from build123d import *

# Parameters (mm, degrees)
SKETCH_R          = 11
PAD_DEPTH         = 5
SKETCH001_R       = 11
PAD001_DEPTH      = 3
SKETCH002_R       = 4.2
PAD002_DEPTH      = 8
SKETCH003_W       = 25.13587
SKETCH003_H       = 8
POCKET_DEPTH      = 11.001
POCKET_DEPTH_BACK = -11.001


with BuildPart() as part:
    # Sketch → Pad (new body)
    with BuildSketch(Plane.XY):
        Circle(SKETCH_R)
        with BuildLine():
            ThreePointArc((-2.683282, 3.1), (0, -4.1), (2.683282, 3.1))
            Line((2.683282, 3.1), (-2.683282, 3.1))
        make_face(mode=Mode.SUBTRACT)
    extrude(amount=-PAD_DEPTH)

    # Sketch001 → Pad001 (join)
    with BuildSketch(Plane.XY.offset(3)):
        Circle(SKETCH001_R)
    extrude(amount=-PAD001_DEPTH)

    # Sketch002 → Pad002 (join)
    with BuildSketch(Plane.XY.offset(11)):
        with Locations((0, 4)):
            Circle(SKETCH002_R)
    extrude(amount=-PAD002_DEPTH)

    # Sketch003 → Pocket (cut, two sides)
    with BuildSketch(Plane.XZ) as pocket_sk:
        with Locations((0.504129, -1)):
            Rectangle(SKETCH003_W, SKETCH003_H)
    extrude(amount=-POCKET_DEPTH, mode=Mode.SUBTRACT)
    extrude(pocket_sk.sketch, amount=-POCKET_DEPTH_BACK, mode=Mode.SUBTRACT)


solid = part.part
Part model, mm, in its own coordinate system. Give positions to 0.01 mm unless a question says otherwise; leave off trailing zeros. Order: outer loops, then holes, each group sorted by start corner. A loop starts at its lowest first (then second) coordinate and runs counter-clockwise, first axis right, second up. Notation, with made-up numbers: (47.5, 28.25) - (73.5, 28.25) arc R19 ccw to (73.5, 63.25) - close; hole circle Ø8 at (58, -18.5). An arc over 180 degrees is marked (long way). Use a Markdown table: item, result.
1) Probe L1, parallel to X at y = 6, z = 5.75; L2, parallel to X at y = 3.5, z = 7.5; L3, parallel to Y at x = -3.25, z = 7.5. List the from-to ranges inside material, lowest first. Write a range as from..to.
Checked values:
| item | result |
|---|---|
| L1 | -3.69..3.69 |
| L2 | -4.17..4.17 |
| L3 | 1.34..6.66 |
2) Flat gauge pins, fed straight in: P1, Ø2, axis at y = 6.5, z = 10, coming from the -X side; P2, Ø4, axis at x = -2.5, z = 5.5, coming from the +Y side. Where does each tip first touch, or does it go through?
Checked values:
| item | result |
|---|---|
| P1 | x = -3.92 |
| P2 | y = 8.17 |
3) Saw through at C-C on y = 6. List the corners of the cut face in (x, z).
Checked values:
| item | result |
|---|---|
| outline | (-3.69, 3) - (3.69, 3) - (3.69, 11) - (-3.69, 11) - close |
4) Saw through at A-A on x = 3.25. List the corners of the cut face in (y, z), plus the area to 3 significant figures.
Checked values:
| item | result |
|---|---|
| outline | (1.34, 3) - (6.66, 3) - (6.66, 11) - (1.34, 11) - close |
| area | 42.6 mm² |
5) Saw through at B-B on z = 9. List the corners of the cut face in (x, y), plus the area to 3 significant figures.
Checked values:
| item | result |
|---|---|
| outline | circle Ø8.4 at (0, 4) |
| area | 55.4 mm² |
